Input: part model. Units: mm. Frame: model coordinates. Coordinates: 2 decimals unless noted, no trailing zeros. Loops run counter-clockwise (first coordinate to the right, second up) from the corner with the lowest first, then second, coordinate; pieces in that order, holes last. Notation, with made-up numbers: (50.5, -7) - (80.5, -7) arc R13 ccw to (80.5, 5) - close; hole circle Ø9 at (-5, -19.5). An arc over 180 degrees is marked (long way). Use one line per item in the form item = value.
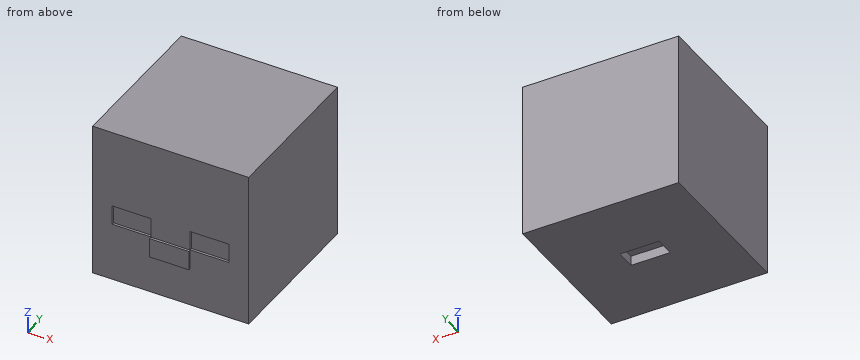
from build123d import *

# Parameters (mm, degrees)
F0_W     = 64
F0_H     = 64
F1_DEPTH = 64
F2_W     = 16
F2_H     = 8
F3_DEPTH = 1
F4_DEPTH = 1
F5_W     = 16.1
F5_H     = 8.1
F6_DEPTH = 4


with BuildPart() as f1:
    # F0 (on Top) → F1 (new body)
    with BuildSketch(Plane.XY):
        Rectangle(F0_W, F0_H)
    extrude(amount=F1_DEPTH)

    # F2 (on face) → F3 (join)
    with BuildSketch(Plane.XZ.offset(32)):
        with Locations((0, 19.9)):
            Rectangle(F2_W, F2_H)
    extrude(amount=F3_DEPTH)

    # F2 (on face) → F4 (cut)
    with BuildSketch(Plane.XZ.offset(32)):
        with Locations((-16, 28)):
            Rectangle(F2_W, F2_H)
        with Locations((16, 28)):
            Rectangle(F2_W, F2_H)
    extrude(amount=-F4_DEPTH, mode=Mode.SUBTRACT)

    # F5 (on face) → F6 (cut)
    with BuildSketch(Plane(origin=(0, 0, 0), x_dir=(1, 0, 0), z_dir=(0, 0, -1))):
        Rectangle(F5_W, F5_H)
    extrude(amount=-F6_DEPTH, mode=Mode.SUBTRACT)


solid = f1.part
Q1. Cut plane C-C, the plane y = -1. Return loops of the section in (x, z).
Check values:
outline = (-32, 0) - (-8.05, 0) - (-8.05, 4) - (8.05, 4) - (8.05, 0) - (32, 0) - (32, 64) - (-32, 64) - close
Q2. Ray query, line 1 along X through (y, z) = (-0.5, 3.5); line 2 along Y through (x, z) = (3.5, 10); line 3 along Y through (x, z) = (-10, 28.5). Return the intervals inside material, ascending. Write a range as [from, to].
Check values:
line_1 = [-32, -8.05], [8.05, 32]
line_2 = [-32, 32]
line_3 = [-31, 32]
Q3. Cut plane B-B, the plane z = 31. Return loops of the section in (x, y).
Check values:
outline = (-32, -32) - (-24, -32) - (-24, -31) - (-8, -31) - (-8, -32) - (8, -32) - (8, -31) - (24, -31) - (24, -32) - (32, -32) - (32, 32) - (-32, 32) - close
Q4. Cut plane A-A, the plane x = 3.5. Return loops of the section in (y, z).
Check values:
outline = (-33, 15.9) - (-32, 15.9) - (-32, 0) - (-4.05, 0) - (-4.05, 4) - (4.05, 4) - (4.05, 0) - (32, 0) - (32, 64) - (-32, 64) - (-32, 23.9) - (-33, 23.9) - close
Q5. First-contact query: P1, Ø0.5, axis at y = -32.5, z = 19, coming from the +X side; P2, Ø2.5, axis at x = 12.5, z = 27.5, coming from the -Y side. Flat tips, straight axial feed; report the tip coordinate or a pass-through.
Check values:
P1 = 8
P2 = -31
Q6. Cut plane D-D, the plane x = 19. Return loops of the section in (y, z), then the cut area to 3 significant figures.
Check values:
outline = (-32, 0) - (32, 0) - (32, 64) - (-32, 64) - (-32, 32) - (-31, 32) - (-31, 24) - (-32, 24) - close
area = 4,090 mm²
